Could you check a few things on this model? Use its own coordinates, in mm. A direction names the side the tool comes from. Coordinates: 2 decimals unless noted, no trailing zeros. Order: outer loops, then holes, each group sorted by start corner. A loop starts at its lowest first (then second) coordinate and runs counter-clockwise, first axis right, second up. Notation, with made-up numbers: (4.5, 57.25) -> (46.5, 57.25) arc R31 cw to (46.5, 92.25) -> close; hole circle Ø9 at (13.25, 63). An arc over 180 degrees is marked (long way). Put each result on its own line as item: value. Start each with the question number.
Q1. If we section it at A-A (y = 0): Please give me the cut outline in (x, z) (3 decimals), and give its area (3 significant figures).
Q2. Will these pins go through, and if not, where does the flat tip stop? pin 1 (2 mm diameter, centred on y = 6.5, z = 3.5, fed in from -X); pin 2 (2 mm diameter, centred on y = 1.5, z = 7.5, fed in from +X); pin 3 (11.5 mm diameter, centred on x = 0, y = 0, fed in from -Z) (3 decimals); pin 4 (4 mm diameter, centred on y = 0, z = 0, fed in from +X).
Q3. For faces 1 (the face through (0, 0, 9.525)), 2 (the face through (11, 0, -15.875)), which set-ups out of +Z, -Z, +X, -X, +Y, -Y let a thin tool reach every point of the face, with its end or its side?
Q4. We'd pull the mould along Y, two halves only. Please class faces 3 (the face through (10.81, 3.03, 0.95)), 4 (the face through (-11, 0, -15.875)), 5 (the face through (5.86, -11.267, -0.422)): +Y half, -Y half, draft (parallel to the pull), parting line (faces both ways), or undercut.
Q5. If we section it at B-B (z = 1): Please give me the cut outline in (x, y) (3 decimals).
Q6. Please list where these lines run through material, in increasing order: line 1 along Z through (x, y) = (-11, 0) (3 decimals); line 2 along X through (y, z) = (6, 9); line 3 along Y through (x, z) = (-3.75, 1).
Q7. If we section it at D-D (z = 8.5): Please give me the cut outline in (x, y) (3 decimals).
Q8. If we section it at C-C (x = 0): Please give me the cut outline in (y, z) (3 decimals), and give its area (3 significant figures).
from build123d import *

# Parameters (mm, degrees)
F0_R          = 12.7
F1_DEPTH      = 15.875
F1_DEPTH_BACK = 15.875
F2_R          = 9.525
F3_DEPTH      = 25.4
F4_R          = 1.27
F6_DEPTH      = 25.4
F6_DEPTH_BACK = 25.4
F7_R          = 3.175
F8_DEPTH      = 12.7
F8_DEPTH_BACK = 12.7


with BuildPart() as f1:
    # F0 (on Top) → F1 (new body, two sides)
    with BuildSketch(Plane.XY) as f1_sk:
        Circle(F0_R)
    extrude(amount=F1_DEPTH)
    extrude(f1_sk.sketch, amount=-F1_DEPTH_BACK)

    # F2 (on face) → F3 (cut)
    with BuildSketch(Plane(origin=(0, 0, -15.875), x_dir=(1, 0, 0), z_dir=(0, 0, -1))):
        Circle(F2_R)
    extrude(amount=-F3_DEPTH, mode=Mode.SUBTRACT)

    # F4
    f4_edges = [f1.edges().sort_by_distance(p)[0] for p in [
        (-12.7, 0, 15.875),
    ]]
    fillet(f4_edges, radius=F4_R)

    # F5 (on Front) → F6 (cut, two sides)
    with BuildSketch(Plane.XZ) as f6_sk:
        with BuildLine():
            ThreePointArc((0, -7.0470880032), (-6.7351920908, -23.307280094), (9.525, -16.5720880032))
            ThreePointArc((9.525, -16.5720880032), (6.7351920908, -9.8368959124), (0, -7.0470880032))
        make_face()
    extrude(amount=F6_DEPTH, mode=Mode.SUBTRACT)
    extrude(f6_sk.sketch, amount=-F6_DEPTH_BACK, mode=Mode.SUBTRACT)

    # F7 (on Right) → F8 (cut, two sides)
    with BuildSketch(Plane.YZ) as f8_sk:
        Circle(F7_R)
    extrude(amount=-F8_DEPTH, mode=Mode.SUBTRACT)
    extrude(f8_sk.sketch, amount=F8_DEPTH_BACK, mode=Mode.SUBTRACT)


solid = f1.part
The answers:
1. outline: (-12.7, -15.875) -> (-9.525, -15.875) -> (-9.525, -3.175) -> (-12.7, -3.175) -> close; (-12.7, 3.175) -> (-9.525, 3.175) -> (-9.525, 9.525) -> (9.525, 9.525) -> (9.525, 3.175) -> (12.7, 3.175) -> (12.7, 14.605) arc R1.27 ccw to (11.43, 15.875) -> (-11.43, 15.875) arc R1.27 ccw to (-12.7, 14.605) -> close; (9.525, -15.875) -> (12.7, -15.875) -> (12.7, -3.175) -> (9.525, -3.175) -> close
1. area: 282 mm^2
2. pin 1: x = -11.45
2. pin 2: x = 12.69
2. pin 3: z = 9.525
2. pin 4: through
3. face 1: -Z
3. face 2: -Z, +X, -X, +Y, -Y
4. face 3: undercut
4. face 4: draft
4. face 5: parting line
5. outline: (-12.337, -3.013) arc R12.7 ccw to (12.337, -3.013) -> (9.036, -3.013) arc R9.525 cw to (-9.036, -3.013) -> close; (-12.337, 3.013) -> (-9.036, 3.013) arc R9.525 cw to (9.036, 3.013) -> (12.337, 3.013) arc R12.7 ccw to start
6. line 1: -15.875 to -3.175, 3.175 to 15.875
6. line 2: -11.19 to -7.4, 7.4 to 11.19
6. line 3: -12.13 to -8.76, 8.76 to 12.13
7. outline: circle Ø25.4 at (0, 0); hole circle Ø19.05 at (0, 0)
8. outline: (-12.7, -7.047) -> (-9.525, -7.047) -> (-9.525, 9.525) -> (9.525, 9.525) -> (9.525, -7.047) -> (12.7, -7.047) -> (12.7, 14.605) arc R1.27 ccw to (11.43, 15.875) -> (-11.43, 15.875) arc R1.27 ccw to (-12.7, 14.605) -> close
8. area: 266 mm^2
